```python
from build123d import *

# Parameters (mm, degrees)
BOSS_EXTRUDE1_DEPTH = 234.95
FILLET1_R           = 0.79375


with BuildPart() as part:
    # Sketch1 → Boss-Extrude1 (new body)
    with BuildSketch(Plane(origin=(0, 0, 0), x_dir=(0, 0, -1), z_dir=(1, 0, 0))):
        Polygon((0, 0), (76.2, 0), (71.617282238, 7.9375), (4.506031045, 7.9375), (0, 3.175), align=None)
    extrude(amount=-BOSS_EXTRUDE1_DEPTH)

    # Fillet1
    fillet1_edges = [part.edges().sort_by_distance(p)[0] for p in [
        (-117.475, 3.175, 0),
        (-117.475, 7.9375, -4.506031045),
        (-117.475, 7.9375, -71.617282238),
        (-117.475, 0, -76.2),
    ]]
    fillet(fillet1_edges, radius=FILLET1_R)


solid = part.part
```
Verification items for the finished model (mm, model axes). Round coordinates to 2 decimals unless told otherwise and drop trailing zeros. Order: outer loops, then holes, each group sorted by start corner. A loop starts at its lowest first (then second) coordinate and runs counter-clockwise, first axis right, second up. Notation, with made-up numbers: (73.25, -13.75) -> (113.25, -13.75) arc R4 ccw to (113.25, -6.75) -> close; hole circle Ø1 at (23, 27). An arc over 180 degrees is marked (long way). Put each result on its own line as item: value. Start each with the question number.
(1) Material ranges on line 1 along Z through (x, y) = (-80.5, 1); line 2 along Z through (x, y) = (-39, 6.75), recorded low to high.
(2) Depth check by flat-ended pin: pin 1 Ø1.5 at (x, y) = (-60.5, 7) entering from -Z; pin 2 Ø1 at (x, y) = (-132, 2.5) entering from -Z. Enter the tip coordinate at first touch or a pass-through.
(3) Section check A-A (x = -59.5). Enter the section's corners in (y, z), then the cut area to 3 significant figures.
(4) Section check B-B (y = 5.5). Enter the section's corners in (x, z), then the cut area to 3 significant figures.
Completed:
1. line 1: z = -75.59 to 0
1. line 2: z = -72.3 to -3.38
2. pin 1: stops at z = -72.59
2. pin 2: stops at z = -75.05
3. outline: (0, -74.83) arc R0.79 ccw to (1.19, -75.51) -> (7.54, -71.85) arc R0.79 ccw to (7.94, -71.16) -> (7.94, -4.85) arc R0.79 ccw to (7.69, -4.27) -> (3.4, -0.22) arc R0.79 ccw to (2.86, 0) -> (0, 0) -> close
3. area: 575 mm2
4. outline: (-234.95, -73.02) -> (0, -73.02) -> (0, -2.2) -> (-234.95, -2.2) -> close
4. area: 16,600 mm2
